Design review of the part shown in the three views and the two pictorial views. Dimensions are in mm from the part's minimum x, y and z. Coordinates: 2 decimals unless noted, no trailing zeros. Loops run counter-clockwise (first coordinate to the right, second up) from the corner with the lowest first, then second, coordinate; pieces in that order, holes last. Notation, with made-up numbers: M -5,-25 L 44,-25 A16 ccw 44,-5 Z; hole C -1.75,52 d11. An arc over 180 degrees is marked long. Use CSV: the item, a comma, the result in double quotes. Start each with the question number.
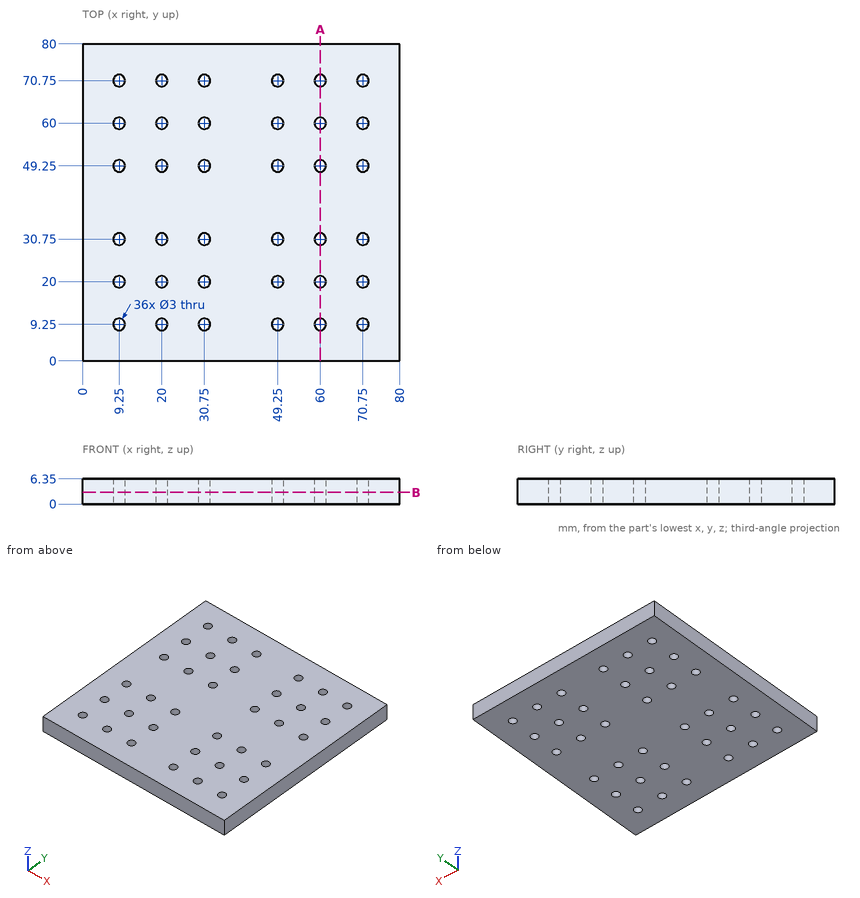
1. Add section A-A (x = 60). Write out the cut boundary in (y, z), plus the area to 3 significant figures.
2. Add section B-B (z = 3). Give the number of separate pieces and of enclosed holes in the cut face, plus the area to 3 significant figures.
3. Insertion check: pin 1 Ø1 at (x, y) = (60.5, 69) entering from -Z. The pin has a flat end and moves straight along its axis. Give the tip position at first contact, or say it passes through.
Solved:
1,outline,"M 0,0 L 7.75,0 L 7.75,6.35 L 0,6.35 Z; M 10.75,0 L 18.5,0 L 18.5,6.35 L 10.75,6.35 Z; M 21.5,0 L 29.25,0 L 29.25,6.35 L 21.5,6.35 Z; M 32.25,0 L 47.75,0 L 47.75,6.35 L 32.25,6.35 Z; M 50.75,0 L 58.5,0 L 58.5,6.35 L 50.75,6.35 Z; M 61.5,0 L 69.25,0 L 69.25,6.35 L 61.5,6.35 Z; M 72.25,0 L 80,0 L 80,6.35 L 72.25,6.35 Z"
1,area,"394 mm^2"
2,separate pieces,"1"
2,enclosed holes,"36"
2,area,"6,150 mm^2"
3,pin 1,"stops at z = 0"
